CAD build for the part. Positions are in the model's coordinates, mm. A direction names the side the tool comes from. Coordinates: 2 decimals unless noted, no trailing zeros. Write item = value, one per line. Start each with the question number.
(1) Tool access for faces 1 (the face through (0, -3.1, 3.8)), 2 (the face through (1.5, -3, 0)), 3 (the face through (0, -3.1, -3.8)), 4 (the face through (-1.5, -1.08, -0.07)), 5 (the face through (1.08, 0.99, 4.88)): list every direction of +Z, -Z, +X, -X, +Y, -Y with a clear straight run to the whole face (end or side of a thin tool).
(2) Flat gauge pins, fed straight in: P1, Ø0.9, axis at x = -0.5, z = -2.5, coming from the +Y side; P2, Ø6, axis at y = 62, z = -3.5, coming from the +X side; P3, Ø3, axis at x = -2.5, z = -1, coming from the +Y side. Where does each tip first touch, or does it go through?
(3) Drill centre lines: line 1 (Y direction, x = 1, z = -2.25); line 2 (Y direction, x = 1.75, z = -0.5); line 3 (Y direction, x = 4, z = 0.25). Where is each one in solid material? Low to high. Write a range as from..to.
(4) Pull direction Y, two halves, no side cores. Call faces 6 (the face through (1.2, 0, 1.2)), 7 (the face through (-1.5, -3, 0)), 8 (the face through (0, -4, 0)): +Y half, -Y half, draft (parallel to the pull), parting line (faces both ways), or undercut.
Autodesk Inventor part; units mm, degrees
ref_plane "YZ Plane" through (0, 0, 0) normal (1, 0, 0) x (0, 1, 0)
ref_plane "XZ Plane" through (0, 0, 0) normal (0, 1, 0) x (-1, 0, 0)
ref_plane "XY Plane" through (0, 0, 0) normal (0, 0, 1) x (1, 0, 0)
sketch "Sketch1" plane through (0, 0, 0) normal (0, 1, 0) x (-1, 0, 0)
  circle A0 centre (0, 0) radius 5
  dimension "d0" = 10
extrude "Extrusion1" add sketch "Sketch1" along normal blind 2
sketch "Sketch2" plane through (0, 0, 0) normal (0, -1, 0) x (1, 0, 0)
  circle A0 centre (0, 0) radius 5
  circle A1 centre (0, 0) radius 1.5
  dimension "d3" = 3
extrude "Extrusion2" add sketch "Sketch2" along normal blind 2.2 contours A1
sketch "Sketch3" plane through (0, -2.2, 0) normal (0, -1, 0) x (1, 0, 0)
  circle A0 centre (0, 0) radius 1.5
  line L0 (-1.5, 3.4914) -> (-1.5, -3.4914)
  line L1 (1.5, 3.4914) -> (1.5, -3.4914)
  line L2 (0, 15.7328) -> (0, -15.032) construction
  circle A1 centre (0, 0) radius 5 construction
  arc A2 (-2, 4.5826) -> (-2, -4.5826) centre (0, 0) ccw construction
  arc A3 (2, -4.5826) -> (2, 4.5826) centre (0, 0) ccw construction
  arc A4 (1.5, 3.4914) -> (-1.5, 3.4914) centre (0, 0) ccw
  arc A5 (-1.5, -3.4914) -> (1.5, -3.4914) centre (0, 0) ccw
  dimension "d13" = 3.8
  dimension "d19" = 3.8
extrude "Extrusion3" add sketch "Sketch3" along normal blind 1.8
fillet "Fillet2" radius 0.8 4 edges at (-1.5, -3.1, 3.4914) (1.5, -3.1, 3.4914) (-1.5, -3.1, -3.4914) (1.5, -3.1, -3.4914)
ref_plane "Work Plane1" through (0, -2.2, 1.5) normal (1, 0, 0) x (0, 0, -1)
sketch "Sketch8" plane through (0, -2.2, 1.5) normal (1, 0, 0) x (0, 0, -1)
  line L0 (-2.3, -1.8) -> (27.7, -1.8) construction
  line L1 (-62.7924, 4.2) -> (54.2342, 4.2) construction
  line L2 (6.5, 2.2) -> (6.5, -147.8) construction
  arc A0 (6.5, 4.2) -> (3, 8.9697) centre (1.5, 4.2) ccw
  line L3 (-2.3, -1.8) -> (-1.9914, -1.8)
  line L4 (3, 8.9697) -> (3, 4.2)
  line L5 (3, 4.2) -> (6.5, 4.2)
  line L6 (-3.5, 2.2) -> (6.5, 2.2)
  line L7 (1.5, 2.2) -> (11.5, 2.2) construction
  line L8 (1.5, 4.2) -> (3, 4.2)
  line L9 (3, 4.2) -> (3, 103.9697)
  line L10 (1.5, 104.2) -> (1.5, 4.2)
  line L11 (1.5, 2.2) -> (1.5, 201.2325) construction
  arc A1 (1.5, 94.2) -> (1.5, 104.2) centre (1.5, 99.2) ccw
  line L12 (1.5, 104.2) -> (1.5, 94.2) construction
  line L13 (3, 103.9697) -> (1.5, 104.2)
  line L14 (1.5, 104.2) -> (1.5, 94.2)
  line L15 (1.5, -218.6065) -> (1.5, 270.0391)
  point P0 (37.0288, 0)
  point P1 (-2.1951, -1.8)
  dimension "d54" = 30
  dimension "d58" = 6
  dimension "d61" = 150
  dimension "d64" = 0
  dimension "d65" = 1.5
  dimension "d66" = 100
  dimension "d68" = 5
  dimension "d70" = 5
revolve "Revolution4" add sketch "Sketch8" angle 360 about axis through (0, 2, 0) along (0, 1, 0)
equation "\"d0\" = HeadConnectorOuterSize"
equation "\"d1\" = EarConnectorHeight"
equation "\"d3\" = HeadConnectorWidth - HeadConnectorTolerance"
equation "\"d4\" = HeadConnectorOuterHeight + HeadConnectorTolerance"
equation "\"d13\" = 0.5 * HeadConnectorDiam - HeadConnectorTolerance"
equation "\"d19\" = 0.5 * HeadConnectorDiam - HeadConnectorTolerance"
equation "\"d10\" = HeadConnectorHeight - HeadConnectorTolerance"
equation "\"d20\" = 0.2 * HeadConnectorProportion"
equation "\"d58\" = HeadConnectorOuterHeight + HeadConnectorHeight + EarConnectorHeight"
equation "\"d65\" = 0.5 * EarWidth"
equation "\"d66\" = EarHeight"
equation "\"d68\" = 0.5 * HeadConnectorOuterSize"
equation "\"d70\" = 0.5 * EarBallSize"
equation "\"EarHeight\" = 100"
equation "\"EarWidth\" = 3"
properties part number "EarShapeET"
Findings below:
q1.face_1 = +Z, -Y
q1.face_2 = +Z, -Z, +X, -Y
q1.face_3 = -Z, -Y
q1.face_4 = none
q1.face_5 = +Y, -Y
q2.P1 = 101.54
q2.P2 = 1.41
q2.P3 = 101.86
q3.line_1 = -4..-2.2, 0..6.35, 92.65..101.35
q3.line_2 = 0..6.66, 92.34..101.66
q3.line_3 = 0..4.99, 94.01..99.99
q4.face_6 = undercut
q4.face_7 = draft
q4.face_8 = -Y half
